from build123d import *

# Parameters (mm, degrees)
SKETCH4_R           = 1.25
SKETCH4_R_2         = 1.5
SKETCH4_W           = 6
SKETCH4_H           = 4
BOSS_EXTRUDE1_DEPTH = 5
FILLET2_R           = 2


with BuildPart() as part:
    # Sketch4 → Boss-Extrude1 (new body)
    with BuildSketch(Plane(origin=(0, 0, 0), x_dir=(1, 0, 0), z_dir=(0, 1, 0))):
        with BuildLine():
            Line((67.306888039, -98.001348092), (-67.306888039, -98.001348092))
            ThreePointArc((-67.306888039, -98.001348092), (-74.37795585, -95.072415903), (-77.306888039, -88.001348092))
            Line((-77.306888039, -88.001348092), (-77.306888039, -38.001348092))
            ThreePointArc((-77.306888039, -38.001348092), (-74.37795585, -30.93028028), (-67.306888039, -28.001348092))
            Line((-67.306888039, -28.001348092), (-38.78630833, -28.001348092))
            ThreePointArc((-38.78630833, -28.001348092), (-32.105125256, -25.441898658), (-28.843972229, -19.073706639))
            Line((-28.843972229, -19.073706639), (-22.256841696, 41.998651908))
            Line((-22.256841696, 41.998651908), (-75.132576553, 37.372624533))
            ThreePointArc((-75.132576553, 37.372624533), (-76.658068454, 37.890459255), (-77.306888039, 39.365013929))
            Line((-77.306888039, 39.365013929), (-77.306888039, 62.182396927))
            Line((-77.306888039, 62.182396927), (-60, 71.998651908))
            Line((-60, 71.998651908), (60, 71.998651908))
            Line((60, 71.998651908), (77.306888039, 62.182396927))
            Line((77.306888039, 62.182396927), (77.306888039, 39.365013929))
            ThreePointArc((77.306888039, 39.365013929), (76.658068454, 37.890459255), (75.132576553, 37.372624533))
            Line((75.132576553, 37.372624533), (22.256841696, 41.998651908))
            Line((22.256841696, 41.998651908), (28.843972229, -19.073706639))
            ThreePointArc((28.843972229, -19.073706639), (32.105125256, -25.441898658), (38.78630833, -28.001348092))
            Line((38.78630833, -28.001348092), (67.306888039, -28.001348092))
            ThreePointArc((67.306888039, -28.001348092), (74.37795585, -30.93028028), (77.306888039, -38.001348092))
            Line((77.306888039, -38.001348092), (77.306888039, -88.001348092))
            ThreePointArc((77.306888039, -88.001348092), (74.37795585, -95.072415903), (67.306888039, -98.001348092))
        make_face()
        with Locations(Location((71.306888039, -54.501348092, 0), (0, 0, 270))):
            Circle(SKETCH4_R, mode=Mode.SUBTRACT)
        with Locations(Location((71.306888039, -71.501348092, 0), (0, 0, 270))):
            Circle(SKETCH4_R, mode=Mode.SUBTRACT)
        with Locations(Location((-71.306888039, -71.501348092, 0), (0, 0, 90))):
            Circle(SKETCH4_R, mode=Mode.SUBTRACT)
        with Locations(Location((-71.306888039, -54.501348092, 0), (0, 0, 90))):
            Circle(SKETCH4_R, mode=Mode.SUBTRACT)
        with Locations(Location((-53.526888039, -87.701348092, 0), (0, 0, 270))):
            Circle(SKETCH4_R_2, mode=Mode.SUBTRACT)
        with Locations(Location((-53.526888039, -48.461348092, 0), (0, 0, 270))):
            Circle(SKETCH4_R_2, mode=Mode.SUBTRACT)
        with Locations(Location((-14.216888039, -48.461348092, 0), (0, 0, 270))):
            Circle(SKETCH4_R_2, mode=Mode.SUBTRACT)
        with Locations(Location((-14.216888039, -87.701348092, 0), (0, 0, 270))):
            Circle(SKETCH4_R_2, mode=Mode.SUBTRACT)
        with BuildLine():
            Line((-47.306888039, 59.498651908), (47.306888039, 59.498651908))
            ThreePointArc((47.306888039, 59.498651908), (49.806888039, 56.998651908), (47.306888039, 54.498651908))
            Line((47.306888039, 54.498651908), (-47.306888039, 54.498651908))
            ThreePointArc((-47.306888039, 54.498651908), (-49.806888039, 56.998651908), (-47.306888039, 59.498651908))
        make_face(mode=Mode.SUBTRACT)
        with BuildLine():
            Line((-57.941248655, 53.047423499), (-66.639525671, 48.113867281))
            ThreePointArc((-66.639525671, 48.113867281), (-70.047483979, 49.055047481), (-69.10630378, 52.463005789))
            Line((-69.10630378, 52.463005789), (-60.408026764, 57.396562007))
            ThreePointArc((-60.408026764, 57.396562007), (-57.000068455, 56.455381807), (-57.941248655, 53.047423499))
        make_face(mode=Mode.SUBTRACT)
        with BuildLine():
            Line((57.941248655, 53.047423499), (66.639525671, 48.113867281))
            ThreePointArc((66.639525671, 48.113867281), (70.047483979, 49.055047481), (69.10630378, 52.463005789))
            Line((69.10630378, 52.463005789), (60.408026764, 57.396562007))
            ThreePointArc((60.408026764, 57.396562007), (57.000068455, 56.455381807), (57.941248655, 53.047423499))
        make_face(mode=Mode.SUBTRACT)
        with Locations((0, 40.807207385)):
            Rectangle(SKETCH4_W, SKETCH4_H, mode=Mode.SUBTRACT)
        with Locations((0, -39.192792615)):
            Rectangle(SKETCH4_W, SKETCH4_H, mode=Mode.SUBTRACT)
    extrude(amount=BOSS_EXTRUDE1_DEPTH)

    # Fillet2
    fillet2_edges = [part.edges().sort_by_distance(p)[0] for p in [
        (-22.256841696, 2.5, -41.998651908),
        (-77.306888039, 2.5, -62.182396927),
        (-60, 2.5, -71.998651908),
        (60, 2.5, -71.998651908),
        (77.306888039, 2.5, -62.182396927),
        (22.256841696, 2.5, -41.998651908),
    ]]
    fillet(fillet2_edges, radius=FILLET2_R)


solid = part.part
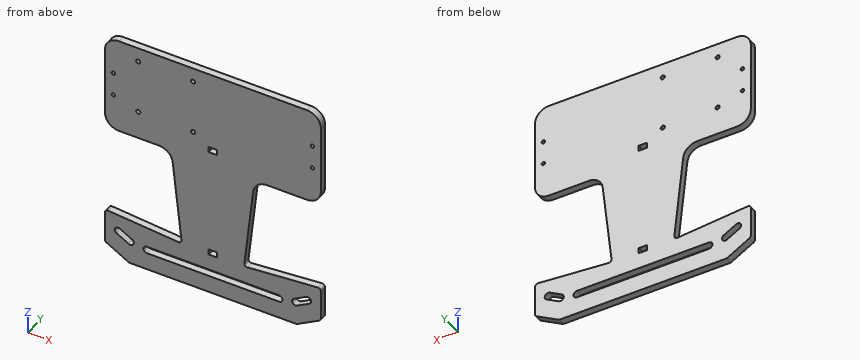
The model under review builds one solid part; all positions refer to its coordinate system, in mm. Coordinates: 2 decimals unless noted, no trailing zeros. Loops run counter-clockwise (first coordinate to the right, second up) from the corner with the lowest first, then second, coordinate; pieces in that order, holes last. Notation, with made-up numbers: (44, 67.25) -> (51, 67.25) arc R21 cw to (51, 97.25) -> close; hole circle Ø7 at (68.5, 8.25). An arc over 180 degrees is marked (long way). Use a Markdown table: item, result. Add a question column.
1. Add section B-B on x = -35.5. Write out the cut boundary in (y, z), plus the area to 3 significant figures.
2. Add section D-D on z = -20. Write out the cut boundary in (x, y), plus the area to 3 significant figures.
3. To check wall thickness, follow line 1 (Z direction, x = -2, y = 3.5); line 2 (Z direction, x = 9, y = 3.7); line 3 (Z direction, x = 40.5, y = 2.1). State the ranges of each line that lie inside material, in increasing order.
4. Add section A-A on x = -5. Write out the cut boundary in (y, z), plus the area to 3 significant figures.
5. Add section C-C on y = 0.9. Give the number of separate pieces and of enclosed holes in the cut face, plus the area to 3 significant figures.
Returned:
| question | item | result |
|---|---|---|
| 1 | outline | (0, -72) -> (5, -72) -> (5, -59.5) -> (0, -59.5) -> close; (0, -54.5) -> (5, -54.5) -> (5, -40.84) -> (0, -40.84) -> close; (0, 27.45) -> (5, 27.45) -> (5, 98) -> (0, 98) -> close |
| 1 | area | 484 mm² |
| 2 | outline | (-24.63, 0) -> (24.63, 0) -> (24.63, 5) -> (-24.63, 5) -> close |
| 2 | area | 246 mm² |
| 3 | line 1 | z = -72 to -59.5, -54.5 to -42.81, -38.81 to 37.19, 41.19 to 98 |
| 3 | line 2 | z = -72 to -59.5, -54.5 to 98 |
| 3 | line 3 | z = -72 to -59.5, -54.5 to -40.4, 28 to 98 |
| 4 | outline | (0, -72) -> (5, -72) -> (5, -59.5) -> (0, -59.5) -> close; (0, -54.5) -> (5, -54.5) -> (5, 98) -> (0, 98) -> close |
| 4 | area | 825 mm² |
| 5 | separate pieces | 1 |
| 5 | enclosed holes | 13 |
| 5 | area | 18,400 mm² |
